For this review, take the finished solid that the model builds, in its own axes (mm). A direction names the side the tool comes from. Give positions to 0.01 mm unless a question says otherwise; leave off trailing zeros. Write each loop counter-clockwise with the first axis right and the second up, starting at its lowest first coordinate (ties: lowest second). Pieces come first, ordered by that corner, then holes. Notation, with made-up numbers: M 83.5,2 L 107.5,2 A21 cw 107.5,24 Z; hole C 63,-10 d1. An arc over 180 degrees is marked long. One line per item, written item: value. Start each with the question number.
Item 1: To check wall thickness, follow probe 1 along Z at (x, y) = (15, -5.5); probe 2 along Y at (x, z) = (-9, 6.25). State the ranges of each line that lie inside material, in increasing order.
Item 2: Consider section C-C, the plane z = 13.25. Write out the cut boundary in (x, y).
Item 3: Mouldability with a two-part tool opening along Y and no side actions: class faces 1 (the face through (-0.74, 7.41, 17.25)), 2 (the face through (-9.25, -23, 12)), 3 (the face through (18.139, 18.098, 0.142)) as released by +Y, released by -Y, zero draft, split by the parting line, or undercut.
Item 4: Clearance check with flat-ended pins moving along their axes: pin 1 Ø2.5 at (x, y) = (-3.5, -21.5) entering from +Z; pin 2 Ø12 at (x, y) = (7, -15.5) entering from +Z; pin 3 Ø1 at (x, z) = (-11.5, 4) entering from -Y. State where each tip first meets the part, or that it passes through.
Item 5: Consider section D-D, the plane y = 5.5. Write out the cut boundary in (x, z).
Item 6: Tool access review of faces 4 (the face through (0, 7, 17.5)), 5 (the face through (18.098, -18.139, 0.142)), 6 (the face through (0, 0, 0)), 7 (the face through (0, -23, 8.5)), 8 (the face through (0.76, 7.33, 17.25)): name each direction out of +Z, -Z, +X, -X, +Y, -Y from which nothing blocks a thin tool from reaching the whole face with its end or side.
Item 7: Consider section A-A, the plane y = -8. Write out the cut boundary in (x, z), and give its area (3 significant figures).
```python
from build123d import *

# Parameters (mm, degrees)
F1_DEPTH = 17
F3_DEPTH = 0.5
F4_DEPTH = 18
F6_R     = 3
F7_SIZE  = 0.5
F8_W     = 18.5
F8_H     = 8
F9_DEPTH = 8


# Not quite as in the source:
# - a fillet or chamfer that OpenCascade refuses, or shapes differently, is made with other operations: its cross-section is extruded or revolved along the edge and cut away or added


with BuildPart() as f1:
    # F0 (on Top) → F1 (new body)
    with BuildSketch(Plane.XY):
        Polygon((-19.25, -19.25), (19.25, -19.25), (19.25, 19.25), (0, 19.25), (-19.25, 19.25), (-19.25, 0), align=None)
        with BuildLine():
            ThreePointArc((-11.75, 0), (-14.75, -3), (-17.75, 0))
            ThreePointArc((-17.75, 0), (-14.75, 3), (-11.75, 0))
        make_face(mode=Mode.SUBTRACT)
        with BuildLine():
            ThreePointArc((3, 14.75), (-2.1213203436, 12.6286796564), (0, 17.75))
            ThreePointArc((0, 17.75), (2.1213203436, 16.8713203436), (3, 14.75))
        make_face(mode=Mode.SUBTRACT)
        with BuildLine():
            ThreePointArc((-11.75, 0), (-14.75, 3), (-17.75, 0))
            ThreePointArc((-17.75, 0), (-14.75, -3), (-11.75, 0))
        make_face()
        with BuildLine():
            ThreePointArc((3, 14.75), (2.1213203436, 16.8713203436), (0, 17.75))
            ThreePointArc((0, 17.75), (-2.1213203436, 12.6286796564), (3, 14.75))
        make_face()
    extrude(amount=F1_DEPTH)

    # F2 (on face) → F3 (join)
    with BuildSketch(Plane.XY.offset(17)):
        Polygon((-1.5, 4.5069497171), (1.5, 4.5069497171), (0, 10.2327093482), align=None)
    extrude(amount=F3_DEPTH)

    # F0 (on Top) → F4 (join)
    with BuildSketch(Plane.XY):
        with BuildLine():
            ThreePointArc((3, 14.75), (2.1213203436, 16.8713203436), (0, 17.75))
            ThreePointArc((0, 17.75), (-2.1213203436, 12.6286796564), (3, 14.75))
        make_face()
        with BuildLine():
            ThreePointArc((-11.75, 0), (-14.75, 3), (-17.75, 0))
            ThreePointArc((-17.75, 0), (-14.75, -3), (-11.75, 0))
        make_face()
    extrude(amount=F4_DEPTH)

    # F5: fillet of radius 2 on 2 edges, made by hand

    # F5_s1 → F5_t2 (revolve, cut)
    with BuildSketch(Plane.YZ):
        with BuildLine():
            ThreePointArc((17.75, 17), (17.0179491924, 17.7320508076), (16.0179491924, 18))
            Line((16.0179491924, 18), (17.75, 18))
            Line((17.75, 18), (17.75, 17))
        make_face()
    revolve(axis=Axis((0, 14.75, 18), (0, 0, 1)), mode=Mode.SUBTRACT)

    # F5_s3 → F5_t4 (revolve, cut)
    with BuildSketch(Plane.XZ):
        with BuildLine():
            ThreePointArc((-17.75, 17), (-17.0179491924, 17.7320508076), (-16.0179491924, 18))
            Line((-16.0179491924, 18), (-17.75, 18))
            Line((-17.75, 18), (-17.75, 17))
        make_face()
    revolve(axis=Axis((-14.75, 0, 18), (0, 0, 1)), mode=Mode.SUBTRACT)

    # F6
    f6_edges = [f1.edges().sort_by_distance(p)[0] for p in [
        (19.25, -19.25, 8.5),
        (-19.25, -19.25, 8.5),
        (-19.25, 19.25, 8.5),
        (19.25, 19.25, 8.5),
    ]]
    fillet(f6_edges, radius=F6_R)

    # F7
    f7_edges = [f1.edges().sort_by_distance(p)[0] for p in [
        (0, 19.25, 17),
        (18.37132, 18.37132, 17),
        (19.25, 0, 17),
        (18.37132, -18.37132, 17),
        (0, -19.25, 17),
        (-18.37132, -18.37132, 17),
        (-19.25, 0, 17),
        (-18.37132, 18.37132, 17),
        (0, -19.25, 0),
        (-18.37132, -18.37132, 0),
        (18.37132, -18.37132, 0),
        (-19.25, 0, 0),
        (19.25, 0, 0),
        (-18.37132, 18.37132, 0),
        (18.37132, 18.37132, 0),
        (0, 19.25, 0),
    ]]
    chamfer(f7_edges, length=F7_SIZE)

    # F8 (on face) → F9 (join)
    with BuildSketch(Plane.XZ.offset(19.25)):
        with Locations((0, 12.5)):
            Rectangle(F8_W, F8_H)
    extrude(amount=F9_DEPTH)


solid = f1.part
```
Model answer:
1. probe 1: z = 0 to 17
1. probe 2: y = -19.25 to 19.25
2. outline: M -19.25,-16.25 A3 ccw -16.25,-19.25 L -9.25,-19.25 L -9.25,-27.25 L 9.25,-27.25 L 9.25,-19.25 L 16.25,-19.25 A3 ccw 19.25,-16.25 L 19.25,16.25 A3 ccw 16.25,19.25 L -16.25,19.25 A3 ccw -19.25,16.25 Z
3. face 1: undercut
3. face 2: zero draft
3. face 3: released by +Y
4. pin 1: stops at z = 16.5
4. pin 2: stops at z = 17
4. pin 3: stops at y = -19.25
5. outline: M -19.25,0.5 L -18.75,0 L 18.75,0 L 19.25,0.5 L 19.25,16.5 L 18.75,17 L 1.24,17 L 1.24,17.5 L -1.24,17.5 L -1.24,17 L -18.75,17 L -19.25,16.5 Z
6. face 4: +Z, +X, -X, -Y
6. face 5: -Z, +X, -Y
6. face 6: -Z, +X, -X, +Y, -Y
6. face 7: -Z, +X, -X, -Y
6. face 8: +Z, +X
7. outline: M -19.25,0.5 L -18.75,0 L 18.75,0 L 19.25,0.5 L 19.25,16.5 L 18.75,17 L -18.75,17 L -19.25,16.5 Z
7. area: 654 mm2
